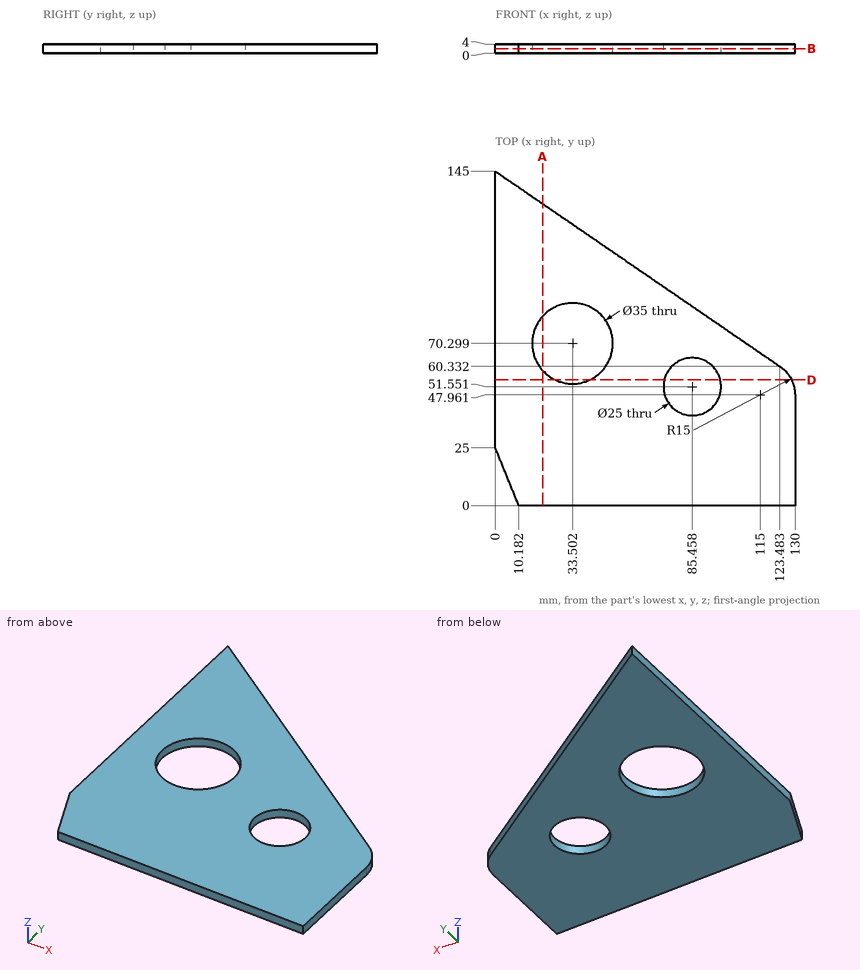
Design review of the part shown in the three views and the two pictorial views. Dimensions are in mm from the part's minimum x, y and z. Coordinates: 2 decimals unless noted, no trailing zeros. Loops run counter-clockwise (first coordinate to the right, second up) from the corner with the lowest first, then second, coordinate; pieces in that order, holes last. Notation, with made-up numbers: M 17.25,66 L 76.25,66 A25 ccw 76.25,92 Z; hole C 73.25,-9.75 d5. An arc over 180 degrees is marked long. Put each result on its own line as item: value. Start each with the question number.
Q1. Add section A-A (x = 20.5). Write out the cut boundary in (y, z), and give its area (3 significant figures).
Q2. Add section B-B (z = 1.95). Write out the cut boundary in (x, y).
Q3. Clearance check with a flat-ended pin moving along its axis: pin 1 (1.5 mm diameter, centred on y = 69, z = 1, fed in from +X) (1 decimal). State where the tip first meets the part, or that it passes through.
Q4. Wall thickness on line 1 (X direction, y = 62.5, z = 1.35) (1 decimal); line 2 (Y direction, x = 39, z = 0.25) (1 decimal); line 3 (X direction, y = 41.5, z = 1.8) (1 decimal): over which ranges is each line inside the solid? List them lowest first.
Q5. Add section D-D (y = 54.5). Write out the cut boundary in (x, z) (1 decimal).
Answers:
1. outline: M 0,0 L 58.59,0 L 58.59,4 L 0,4 Z; M 82.01,0 L 130.94,0 L 130.94,4 L 82.01,4 Z
1. area: 430 mm^2
2. outline: M 0,25 L 10.18,0 L 130,0 L 130,47.96 A15 ccw 123.48,60.33 L 0,145 Z; hole C 33.5,70.3 d35; hole C 85.46,51.55 d25
3. pin 1: stops at x = 111.9
4. line 1: x = 0 to 17.8, 49.2 to 79.4, 91.5 to 120.3
4. line 2: y = 0 to 53.7, 86.9 to 118.3
4. line 3: x = 0 to 78, 92.9 to 130
5. outline: M 0,0 L 26,0 L 26,4 L 0,4 Z; M 41,0 L 73.3,0 L 73.3,4 L 41,4 Z; M 97.6,0 L 128.5,0 L 128.5,4 L 97.6,4 Z
